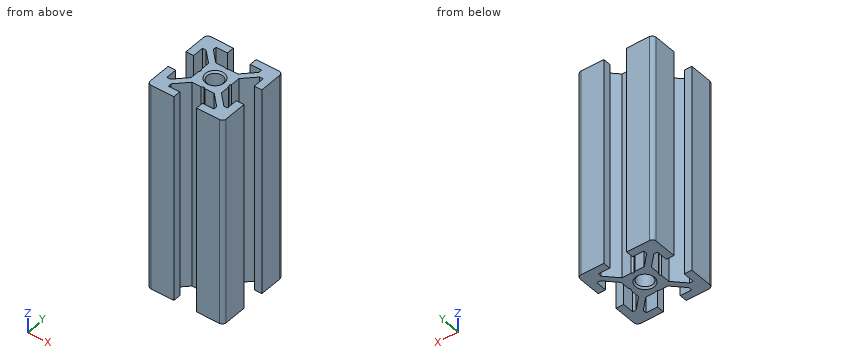
Autodesk Inventor part; units mm, degrees
ref_plane "C1_XY" through (0, 0, 0) normal (0, 0, 1) x (1, 0, 0)
ref_plane "C1_YZ" through (0, 0, 0) normal (1, 0, 0) x (0, 1, 0)
ref_plane "C1_ZX" through (0, 0, 0) normal (0, 1, 0) x (0, 0, 1)
sketch "Sketch_1" plane through (0, 0, 0) normal (0, 0, 1) x (1, 0, 0)
  line L0 (-10, 3) -> (-8, 3)
  line L1 (-8, 3) -> (-8, 6)
  line L2 (-8, 6) -> (-7.0607, 6)
  line L3 (-7.0607, 6) -> (-4, 2.9393)
  line L4 (-4, 2.9393) -> (-4, 0.5196)
  line L5 (-4, 0.5196) -> (-3.7, 0)
  line L6 (-3.7, 0) -> (-4, -0.5196)
  line L7 (-4, -0.5196) -> (-4, -2.9393)
  line L8 (-4, -2.9393) -> (-7.0607, -6)
  line L9 (-7.0607, -6) -> (-8, -6)
  line L10 (-8, -6) -> (-8, -3)
  line L11 (-8, -3) -> (-10, -3)
  line L12 (-10, -3) -> (-10, -9)
  arc A0 (-10, -9) -> (-9, -10) centre (-9, -9) ccw
  line L13 (-9, -10) -> (-3, -10)
  line L14 (-3, -10) -> (-3, -8)
  line L15 (-3, -8) -> (-6, -8)
  line L16 (-6, -8) -> (-6, -7.0607)
  line L17 (-6, -7.0607) -> (-2.9393, -4)
  line L18 (-2.9393, -4) -> (-0.5196, -4)
  line L19 (-0.5196, -4) -> (0, -3.7)
  line L20 (0, -3.7) -> (0.5196, -4)
  line L21 (0.5196, -4) -> (2.9393, -4)
  line L22 (2.9393, -4) -> (6, -7.0607)
  line L23 (6, -7.0607) -> (6, -8)
  line L24 (6, -8) -> (3, -8)
  line L25 (3, -8) -> (3, -10)
  line L26 (3, -10) -> (9, -10)
  arc A1 (9, -10) -> (10, -9) centre (9, -9) ccw
  line L27 (10, -9) -> (10, -3)
  line L28 (10, -3) -> (8, -3)
  line L29 (8, -3) -> (8, -6)
  line L30 (8, -6) -> (7.0607, -6)
  line L31 (7.0607, -6) -> (4, -2.9393)
  line L32 (4, -2.9393) -> (4, -0.5196)
  line L33 (4, -0.5196) -> (3.7, 0)
  line L34 (3.7, 0) -> (4, 0.5196)
  line L35 (4, 0.5196) -> (4, 2.9393)
  line L36 (4, 2.9393) -> (7.0607, 6)
  line L37 (7.0607, 6) -> (8, 6)
  line L38 (8, 6) -> (8, 3)
  line L39 (8, 3) -> (10, 3)
  line L40 (10, 3) -> (10, 9)
  arc A2 (10, 9) -> (9, 10) centre (9, 9) ccw
  line L41 (9, 10) -> (3, 10)
  line L42 (3, 10) -> (3, 8)
  line L43 (3, 8) -> (6, 8)
  line L44 (6, 8) -> (6, 7.0607)
  line L45 (6, 7.0607) -> (2.9393, 4)
  line L46 (2.9393, 4) -> (0.5196, 4)
  line L47 (0.5196, 4) -> (0, 3.7)
  line L48 (0, 3.7) -> (-0.5196, 4)
  line L49 (-0.5196, 4) -> (-2.9393, 4)
  line L50 (-2.9393, 4) -> (-6, 7.0607)
  line L51 (-6, 7.0607) -> (-6, 8)
  line L52 (-6, 8) -> (-3, 8)
  line L53 (-3, 8) -> (-3, 10)
  line L54 (-3, 10) -> (-9, 10)
  arc A3 (-9, 10) -> (-10, 9) centre (-9, 9) ccw
  line L55 (-10, 9) -> (-10, 3)
extrude "Extrusion1" add sketch "Sketch_1" against normal blind 55
sketch "Sketch2" plane through (0, 0, 0) normal (0, 0, 1) x (1, 0, 0)
  point P0 (0, 0)
hole "Hole1" at (0, 0, 0) direction (0, 0, -1) diameter 4.134 depth 15 countersink diameter 5 countersink angle 90
sketch "Sketch3" plane through (0, 0, -55) normal (0, 0, -1) x (-1, 0, 0)
  point P0 (0, 0)
hole "Hole2" at (0, 0, -55) direction (0, 0, 1) diameter 4.134 depth 15 countersink diameter 5 countersink angle 90
sketch "Sketch4" plane through (0, 0, -40) normal (0, 0, -1) x (-1, 0, 0)
  point P0 (0, 0)
hole "Hole3" at (0, 0, -40) direction (0, 0, 1) diameter 4.2 depth 25
ref_plane "C1_XY" through (0, 0, 0) normal (0, 0, 1) x (1, 0, 0)
ref_plane "C1_YZ" through (0, 0, 0) normal (1, 0, 0) x (0, 1, 0)
ref_plane "C1_ZX" through (0, 0, 0) normal (0, 1, 0) x (0, 0, 1)
properties part number "HFSB5-2020-55-TPW"
Could you check a few things on this model? Use its own coordinates, in mm. Coordinates: 2 decimals unless noted, no trailing zeros. Loops run counter-clockwise (first coordinate to the right, second up) from the corner with the lowest first, then second, coordinate; pieces in that order, holes last. Notation, with made-up numbers: M 66,81.5 L 106,81.5 A28 cw 106,116.5 Z; hole C 52,16 d11. An arc over 180 degrees is marked long. Put each result on its own line as item: value. Start each with the question number.
(1) I need wall thicknesses on line 1 (Y direction, x = 0, z = -45.75); line 2 (X direction, y = 3.5, z = -52); line 3 (X direction, y = 5.75, z = -5). Which ranges of each line are inside material? Lowest first, please. Write a range as from..to.
(2) Will these pins go through, and if not, where does the flat tip stop? P1, Ø1.2, axis at x = -1.5, z = -38, coming from the +Y side; P2, Ø0.7, axis at y = 2, z = -21.5, coming from the +X side.
(3) Suppose I cut it at A-A on y = -5.25. Please give me the cut outline in (x, z).
Solutions:
1. line 1: y = -3.7..-2.07, 2.07..3.7
1. line 2: x = -10..-8, -4.56..4.56, 8..10
1. line 3: x = -10..-8, -6.81..-4.69, 4.69..6.81, 8..10
2. P1: stops at y = 4
2. P2: stops at x = 4
3. outline: M -10,-55 L -8,-55 L -8,0 L -10,0 Z; M -6.31,-55 L -4.19,-55 L -4.19,0 L -6.31,0 Z; M 4.19,-55 L 6.31,-55 L 6.31,0 L 4.19,0 Z; M 8,-55 L 10,-55 L 10,0 L 8,0 Z
